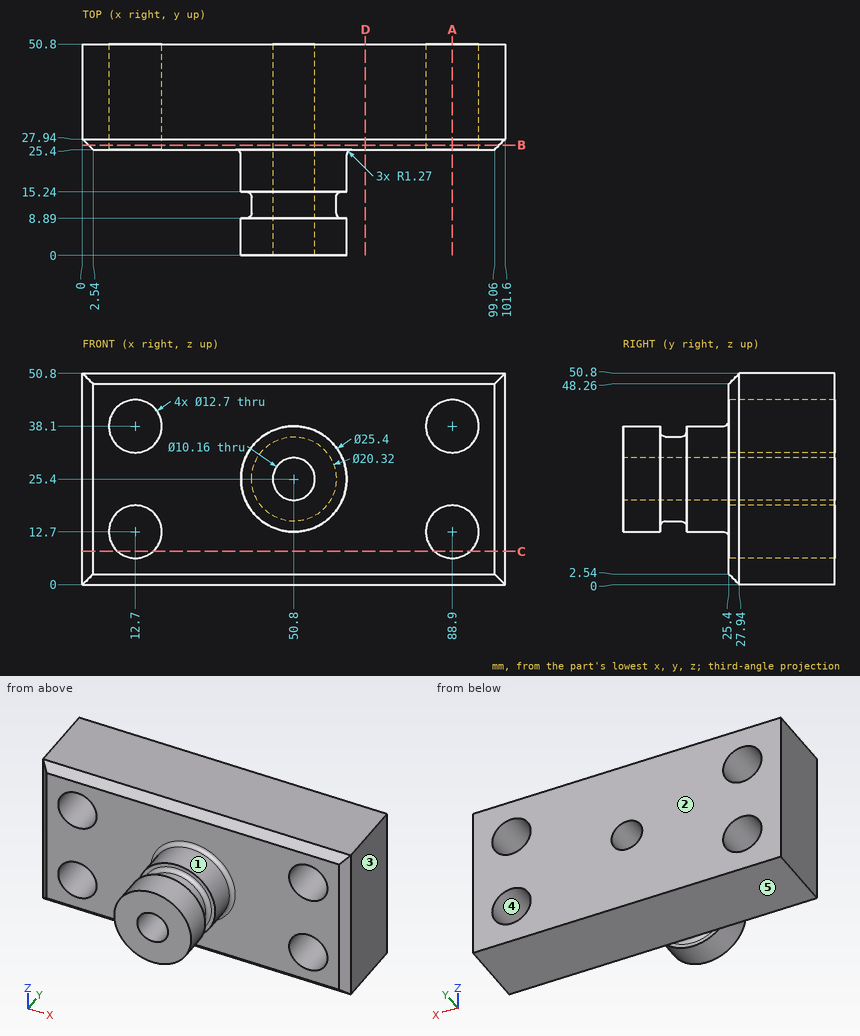
Answer from the drawing. Dimensions are ordinates in mm from the lowest x, y and z of the part. A direction names the side the tool comes from. Round coordinates to 2 decimals unless told otherwise and drop trailing zeros. Write each loop counter-clockwise with the first axis right and the second up, starting at its lowest first coordinate (ties: lowest second). Pieces come first, ordered by that corner, then holes. Notation, with made-up numbers: (58.5, 53.25) -> (68.5, 53.25) arc R21 ccw to (68.5, 73.25) -> close; hole circle Ø3 at (-9.75, 89.5). An arc over 180 degrees is marked (long way). Write each question's results on one line, items separated by ' | '.
1) The part is cut by section B-B (y = 26.5). Write down the section's boundary in (x, z).
Findings:
outline: (1.44, 1.44) -> (100.16, 1.44) -> (100.16, 49.36) -> (1.44, 49.36) -> close; hole circle Ø12.7 at (12.7, 12.7); hole circle Ø12.7 at (12.7, 38.1); hole circle Ø10.16 at (50.8, 25.4); hole circle Ø12.7 at (88.9, 12.7); hole circle Ø12.7 at (88.9, 38.1)
2) Which of the six approach directions +Z, -Z, +X, -X, +Y, -Y give full straight-line access (tool end or side, diameter ignored) to the marked faces 1 and 2?
Findings:
face 1: -Y | face 2: +Z, -Z, +X, -X, +Y
3) For a pull along Z with two mould halves and no side action, classify the marked faces 3, 4 and 5 as +Z half, -Z half, draft (parallel to the pull), parting line (faces both ways), or undercut.
Findings:
face 3: draft | face 4: undercut | face 5: -Z half
4) Consider line 1 along Z through (x, y) = (88, 32); line 2 along Y through (x, z) = (53.5, 46.5); line 3 along X through (y, z) = (13, 24.5). Determine where each line is inside the solid, lowest interval first. Write a range as [from, to].
Findings:
line 1: z = [0, 6.41], [18.99, 31.81], [44.39, 50.8] | line 2: y = [25.4, 50.8] | line 3: x = [40.68, 45.8], [55.8, 60.92]
5) The part is cut by section A-A (x = 88.9). Write down the section's boundary in (y, z), and give its area (3 significant figures).
Findings:
outline: (25.4, 2.54) -> (27.94, 0) -> (50.8, 0) -> (50.8, 6.35) -> (25.4, 6.35) -> close; (25.4, 19.05) -> (50.8, 19.05) -> (50.8, 31.75) -> (25.4, 31.75) -> close; (25.4, 44.45) -> (50.8, 44.45) -> (50.8, 50.8) -> (27.94, 50.8) -> (25.4, 48.26) -> close | area: 639 mm²
6) Flat-ended cylindrical pins translate along their axes: pin 1 (1 mm diameter, centred on y = 11.5, z = 36.5, fed in from +X); pin 2 (2 mm diameter, centred on x = 30, z = 8, fed in from -Y); pin 3 (1.5 mm diameter, centred on y = 11.5, z = 29, fed in from -X); pin 4 (8 mm diameter, centred on y = 7, z = 13, fed in from +X). Find the tip coordinate at first contact, or state that the pin passes through.
Findings:
pin 1: passes through | pin 2: stops at y = 25.4 | pin 3: stops at x = 41.05 | pin 4: stops at x = 60.33
7) The part is cut by section D-D (x = 68). Write down the section's boundary in (y, z), and give its area (3 significant figures).
Findings:
outline: (25.4, 2.54) -> (27.94, 0) -> (50.8, 0) -> (50.8, 50.8) -> (27.94, 50.8) -> (25.4, 48.26) -> close | area: 1,280 mm²
8) The part is cut by section C-C (z = 8). Write down the section's boundary in (x, y), and give its area (3 significant figures).
Findings:
outline: (0, 27.94) -> (2.54, 25.4) -> (8.43, 25.4) -> (8.43, 50.8) -> (0, 50.8) -> close; (16.97, 25.4) -> (84.63, 25.4) -> (84.63, 50.8) -> (16.97, 50.8) -> close; (93.17, 25.4) -> (99.06, 25.4) -> (101.6, 27.94) -> (101.6, 50.8) -> (93.17, 50.8) -> close | area: 2,140 mm²
